```python
from build123d import *

# Parameters (mm, degrees)
BOSS_EXTRUDE1_DEPTH = 152.4
SKETCH3_OUTSIDE_W   = 273.93
SKETCH3_OUTSIDE_H   = 229.576
CUT_EXTRUDE2_DEPTH  = 381.660734008
SHELL1_T            = -6.35
CUT_EXTRUDE3_DEPTH  = 381.660734008


with BuildPart() as part:
    # Sketch2 → Boss-Extrude1 (new body)
    with BuildSketch(Plane(origin=(0, 0, 0), x_dir=(1, 0, 0), z_dir=(0, 1, 0))):
        Polygon((-57.15, 0), (224.536, 0), (-24.357683353, -196.753899884), align=None)
    extrude(amount=BOSS_EXTRUDE1_DEPTH)

    # Sketch3 outside → Cut-Extrude2 (cut, through all)
    with BuildSketch(Plane(origin=(-63.5, 0, 0), x_dir=(0, 0, -1), z_dir=(1, 0, 0))):
        with Locations((-98.377, 76.2)):
            Rectangle(SKETCH3_OUTSIDE_W, SKETCH3_OUTSIDE_H)
        Polygon((0, 152.4), (-152.4, 107.95), (-261.257142857, 76.2), (-152.4, 44.45), (0, 0), align=None, mode=Mode.SUBTRACT)
    extrude(amount=CUT_EXTRUDE2_DEPTH, mode=Mode.SUBTRACT)

    # Shell1
    shell1_openings = [part.faces().sort_by_distance(p)[0] for p in [
        (83.693, 76.2, 0),
    ]]
    offset(amount=SHELL1_T, openings=shell1_openings, kind=Kind.INTERSECTION)

    # Sketch4 → Cut-Extrude3 (cut, through all)
    with BuildSketch(Plane(origin=(-63.5, 0, 0), x_dir=(0, 0, -1), z_dir=(1, 0, 0))):
        Polygon((0, 274.61160546), (-196.753899884, 217.225051327), (-196.753899884, 64.001137466), (0, 6.614583333), align=None)
    extrude(amount=CUT_EXTRUDE3_DEPTH, mode=Mode.SUBTRACT)


solid = part.part
```
Here's how the part is built. I have some questions about the finished solid (model axes, mm). Coordinates: 2 decimals unless noted, no trailing zeros. Write each loop counter-clockwise with the first axis right and the second up, starting at its lowest first coordinate (ties: lowest second). Pieces come first, ordered by that corner, then holes. Notation, with made-up numbers: (66.25, 52.25) -> (86.25, 52.25) arc R23 cw to (86.25, 64.25) -> close; hole circle Ø11 at (61.5, 44). An arc over 180 degrees is marked (long way). Use a Markdown table: item, result. Add a question column.
(1) Please list where these lines run through material, in increasing order: line 1 (Y direction, x = 26, z = 50); line 2 (X direction, y = 26, z = 67); line 3 (Y direction, x = -42.5, z = 59.5).
(2) I'm going to push flat-ended pins straight in: P1, Ø6, axis at x = 59.5, z = 122.5, coming from the +Y side; P2, Ø1, axis at x = 2.5, z = 142.5, coming from the -Y side; P3, Ø10, axis at x = 102, y = 41.5, coming from the +Z side. Where does each tip first touch, or does it pass through?
(3) If we section it at A-A, the plane z = 181.5: Write out the boundary of the cut face in (x, y).
(4) If we section it at B-B, the plane x = 5.5: Write out the boundary of the cut face in (y, z), and give its area (3 significant figures).
Outcome:
| question | item | result |
|---|---|---|
| 1 | line 1 | y = 14.58 to 21.2 |
| 1 | line 2 | x = -45.98 to 139.78 |
| 1 | line 3 | y = 17.35 to 23.97 |
| 2 | P1 | stops at y = 43.22 |
| 2 | P2 | stops at y = 41.42 |
| 2 | P3 | passes through |
| 3 | outline | (-26.9, 52.94) -> (-5.06, 52.94) -> (-5.06, 59.55) -> (-26.9, 59.55) -> close |
| 4 | outline | (0, 0) -> (6.61, 0) -> (57.12, 173.15) -> (50.5, 173.15) -> close |
| 4 | area | 1,150 mm^2 |
